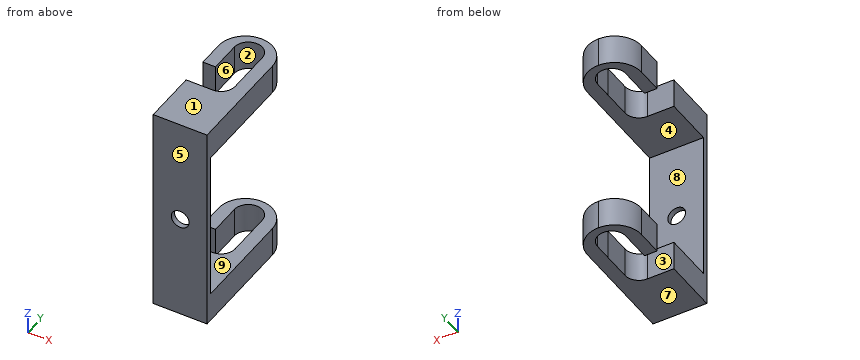
Autodesk Inventor part; units mm, degrees
ref_plane "YZ Plane" through (0, 0, 0) normal (1, 0, 0) x (0, 1, 0)
ref_plane "XZ Plane" through (0, 0, 0) normal (0, 1, 0) x (-1, 0, 0)
ref_plane "XY Plane" through (0, 0, 0) normal (0, 0, 1) x (1, 0, 0)
sketch "Sketch1" plane through (0, 0, 0) normal (0, 1, 0) x (-1, 0, 0)
  line L0 (10, 67.88) -> (-10, 67.88)
  line L1 (-10, 67.88) -> (-10, -10)
  line L2 (-10, -10) -> (10, -10)
  line L3 (10, -10) -> (10, 67.88)
  point P0 (0, 0)
  dimension "d0" = 20
  dimension "d1" = 77.88
extrude "Extrusion1" add sketch "Sketch1" along normal blind 2
sketch "Sketch2" plane through (0, 2, 0) normal (0, 1, 0) x (1, 0, 0)
  line L0 (-10, -67.88) -> (10, -67.88)
  line L1 (0, -67.88) -> (-6.35, -67.88)
  line L2 (-6.35, -56.98) -> (6.35, -56.98)
  line L3 (6.35, -67.88) -> (0, -67.88)
  line L4 (10, 10) -> (-10, 10)
  line L5 (-6.35, -0.9) -> (6.35, -0.9)
  line L6 (-6.35, 10) -> (6.35, 10)
  line L7 (-6.35, -67.88) -> (-10, -67.88)
  line L8 (-10, 10) -> (-10, -67.88)
  line L9 (-10, -56.98) -> (-6.35, -56.98)
  line L10 (6.35, -67.88) -> (10, -67.88)
  line L11 (10, -67.88) -> (10, 10)
  line L12 (10, -56.98) -> (6.35, -56.98)
  line L13 (6.35, -0.9) -> (10, -0.9)
  line L14 (10, 10) -> (6.35, 10)
  line L15 (10, -0.9) -> (10, 10)
  line L16 (10, -67.88) -> (10, -56.98)
  line L17 (-10, -67.88) -> (-10, -56.98)
  line L18 (-6.35, -0.9) -> (-10, -0.9)
  line L19 (-10, -0.9) -> (-10, 10)
  line L20 (-10, 10) -> (-6.35, 10)
  point P0 (0, 0)
  dimension "d4" = 6.35
  dimension "d5" = 10.9
  dimension "d6" = 12.7
  dimension "d7" = 10.9
extrude "Extrusion2" add sketch "Sketch2" along normal blind 48.3354 contours L8 L9 L2 L12 L11 L0 | L8 L4 L11 L13 L5 L18
sketch "Sketch9" plane through (-10, 0, 67.88) normal (0, 0, 1) x (1, 0, 0)
  arc A0 (15.084, 42.3223) -> (4.684, 42.3223) centre (9.884, 42.3223) ccw
  line L0 (15.084, 35.9247) -> (15.084, 42.3223)
  line L1 (4.684, 41.1247) -> (4.684, 42.3223)
  arc A1 (15.084, 42.3223) -> (4.684, 42.3223) centre (9.884, 42.3223) ccw
  line L2 (4.684, 42.3223) -> (4.684, 35.9247)
  line L3 (9.8827, 20.3222) -> (-0.0013, 20.3222)
  line L4 (-0.0013, 30.726) -> (-0.0013, 20.3222)
  line L5 (4.684, 35.9247) -> (4.684, 30.726)
  line L6 (15.084, 35.9247) -> (15.0853, 25.5254)
  arc A2 (15.084, 35.9247) -> (15.084, 35.9251) centre (9.884, 35.9243) ccw
  line L7 (4.684, 30.726) -> (-0.0013, 30.726)
  arc A3 (9.8827, 20.3222) -> (15.0853, 25.5254) centre (9.8827, 25.5248) ccw
  point P0 (10, 0)
fillet "Fillet4" radius 10 4 edges at (10, 50.3354, 62.43) (-10, 50.3354, 62.43) (-10, 50.3354, -4.55) (10, 50.3354, -4.55)
sketch "Sketch10" plane through (0, 2, 0) normal (0, 1, 0) x (1, 0, 0)
  line L0 (10, -67.88) -> (-10, -67.88)
  line L1 (-10, 10) -> (10, 10)
  line L2 (10, -56.98) -> (10, -0.9)
  line L3 (-10, -0.9) -> (-10, -56.98)
  line L4 (10, -28.94) -> (-10, -28.94)
  circle A0 centre (0, -28.94) radius 3.302
  point P0 (0, 0)
  dimension "d53" = 77.88
  dimension "d54" = 6.604
extrude "Extrusion10" cut sketch "Sketch10" against normal blind 2
extrude "Extrusion11" cut sketch "Sketch9" against normal through all
properties part number "6 Backet Adjustment"
The listing builds one solid part. Answer for the finished solid, in the listing's coordinates (mm). Face numbers are marked on the shaded views. A direction names the side the tool comes from. Coordinates: 2 decimals unless noted, no trailing zeros. Order: outer loops, then holes, each group sorted by start corner. A loop starts at its lowest first (then second) coordinate and runs counter-clockwise, first axis right, second up.
Q1. A cutting plane is placed at C-C, the plane y = 16. Write down the section's boundary in (x, z).
Q2. Consider line 1 (Z direction, x = 0, y = 0.85); line 2 (Z direction, x = -5.75, y = 35.5); line 3 (X direction, y = 0.95, z = 28.94). Determine where each line is inside the solid, lowest interval first.
Q3. For a pull along Z with two mould halves and no side action, classify the marked faces 6, 7, 8 and 9 as pulls with the +Z half, pulls with the -Z half, needs draft (parallel to the pull), parting line crosses it, or undercut.
Q4. A cutting plane is placed at B-B, the plane y = 38. Write down the section's boundary in (x, z), and give its area (3 significant figures).
Q5. A cutting plane is placed at A-A, the plane z = 28.94. Write down the section's boundary in (x, y).
Q6. A cutting plane is placed at D-D, the plane x = -2.5. Write down the section's boundary in (y, z).
Q7. Which of the six approach directions +Z, -Z, +X, -X, +Y, -Y give full straight-line access (tool end or side, diameter ignored) to the marked faces 1, 2, 3, 4 and 5?
Q8. Given P1, Ø5, axis at x = -5.5, z = 16.5, coming from the +Y side; P2, Ø3, axis at x = -3.5, z = -4, coming from the +Y side; P3, Ø1.4, axis at x = -7.5, z = 62.5, coming from the -Y side; P4, Ø5, axis at x = -4, z = 62.5, coming from the +Y side, each flat-ended and moving along its own axis, determine where each tip first touches the part or whether it passes through.
Answers follow:
1. outline: (-10, -10) - (10, -10) - (10, 0.9) - (-10, 0.9) - close; (-10, 56.98) - (10, 56.98) - (10, 67.88) - (-10, 67.88) - close
2. line 1: z = -10 to 25.64, 32.24 to 67.88
2. line 2: z = -10 to 0.9, 56.98 to 67.88
2. line 3: x = -10 to -3.3, 3.3 to 10
3. face 6: needs draft
3. face 7: pulls with the -Z half
3. face 8: undercut
3. face 9: undercut
4. outline: (-10, -10) - (-5.32, -10) - (-5.32, 0.9) - (-10, 0.9) - close; (-10, 56.98) - (-5.32, 56.98) - (-5.32, 67.88) - (-10, 67.88) - close; (5.08, -10) - (10, -10) - (10, 0.9) - (5.08, 0.9) - close; (5.08, 56.98) - (10, 56.98) - (10, 67.88) - (5.08, 67.88) - close
4. area: 209 mm2
5. outline: (-10, 0) - (-3.3, 0) - (-3.3, 2) - (-10, 2) - close; (3.3, 0) - (10, 0) - (10, 2) - (3.3, 2) - close
6. outline: (0, -10) - (20.32, -10) - (20.32, 0.9) - (2, 0.9) - (2, 26.78) - (0, 26.78) - close; (0, 31.1) - (2, 31.1) - (2, 56.98) - (20.32, 56.98) - (20.32, 67.88) - (0, 67.88) - close; (46.94, -10) - (50.02, -10) - (50.02, 0.9) - (46.94, 0.9) - close; (46.94, 56.98) - (50.02, 56.98) - (50.02, 67.88) - (46.94, 67.88) - close
7. face 1: +Z, +X, -X, +Y, -Y
7. face 2: +Z, -Z
7. face 3: +Z, -Z, -X
7. face 4: +X, -X, +Y
7. face 5: +Z, -Z, +X, -X, -Y
8. P1: stops at y = 2
8. P2: stops at y = 50.13
8. P3: stops at y = 0
8. P4: stops at y = 50.22
